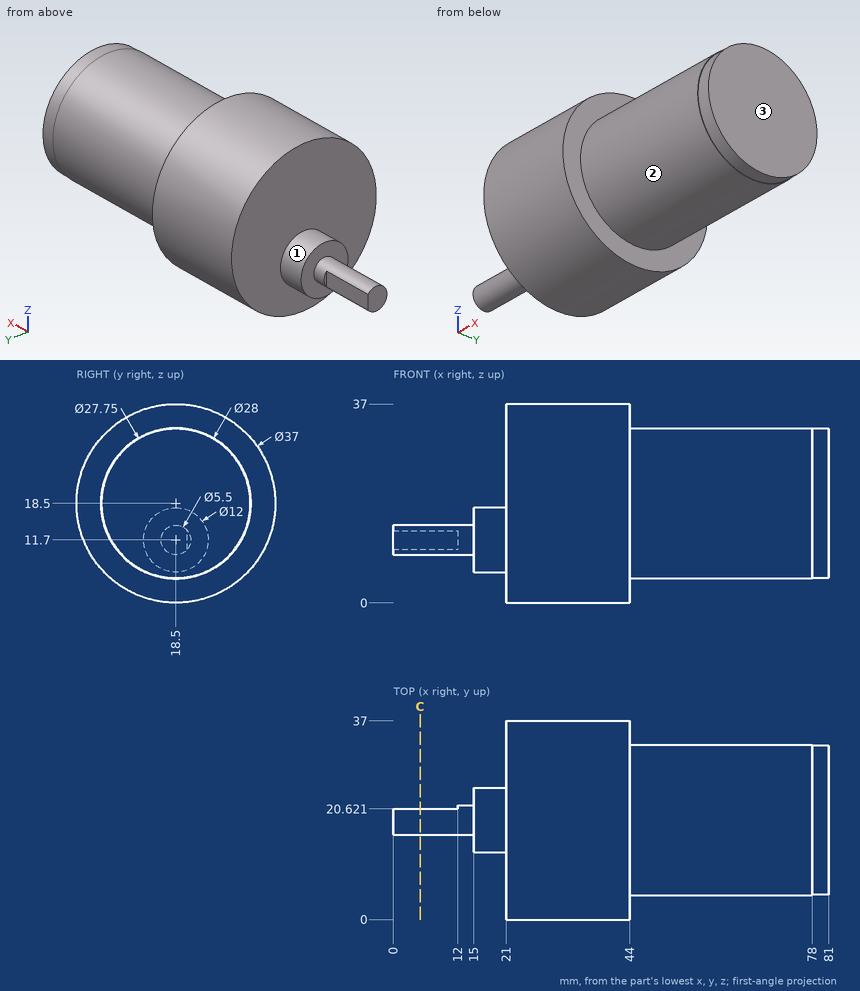
Geometry check sheet. Reference: drawing and pictorial views, mm from the part's lowest x, y, z. A direction names the side the tool comes from. Give positions to 0.01 mm unless a question says otherwise; leave off trailing zeros. Loops run counter-clockwise (first coordinate to the right, second up) from the corner with the lowest first, then second, coordinate; pieces in that order, holes last. Notation, with made-up numbers: (46, -27) -> (67, -27) arc R14 ccw to (67, -6) -> close; hole circle Ø11 at (79.5, 16.5). An arc over 180 degrees is marked (long way). Answer in a Markdown table with one row per item. Add a question column.
1) Gauge pin test, flat ends, axial feed: P1, Ø12, axis at x = 8, y = 5.5, coming from the -Z side; P2, Ø3, axis at x = 68, y = 6.5, coming from the -Z side; P3, Ø3, axis at x = 14, z = 7.5, coming from the +Y side; P4, Ø10, axis at y = 10, z = 17, coming from the -X side. Record the tip position at first contact, or that the pin passes through.
2) Material ranges on probe 1 along Z at (x, y) = (69, 19); probe 2 along X at (y, z) = (13, 34); probe 3 along X at (y, z) = (22.5, 16), recorded low to high. Write a range as from..to.
3) Cross-section at C-C on x = 5. Record the boundary of the cut face in (y, z).
4) Set-up check for the marked faces 1, 2 and 3: record each of +Z, -Z, +X, -X, +Y, -Y from which the full face is reachable in a straight line by a thin tool's end or side.
Outcome:
| question | item | result |
|---|---|---|
| 1 | P1 | passes through |
| 1 | P2 | stops at z = 9.24 |
| 1 | P3 | stops at y = 23.65 |
| 1 | P4 | stops at x = 15 |
| 2 | probe 1 | z = 4.51..32.49 |
| 2 | probe 2 | x = 21..44 |
| 2 | probe 3 | x = 15..81 |
| 3 | outline | (20.62, 9.95) -> (20.62, 13.45) arc R2.75 ccw (long way) to start |
| 4 | face 1 | -X |
| 4 | face 2 | +X |
| 4 | face 3 | +Z, -Z, +X, +Y, -Y |
